Check sheet for the modelled part. Datum: model origin and axes. Units: mm. Face numbers are marked on the shaded views. A direction names the side the tool comes from. Round coordinates to 2 decimals unless told otherwise and drop trailing zeros. Order: outer loops, then holes, each group sorted by start corner. A loop starts at its lowest first (then second) coordinate and runs counter-clockwise, first axis right, second up. Notation, with made-up numbers: (-3, 63) -> (50, 63) arc R29 cw to (50, 89) -> close; hole circle Ø1 at (-22, 18). An arc over 180 degrees is marked (long way). Answer in a Markdown table with one row per item.
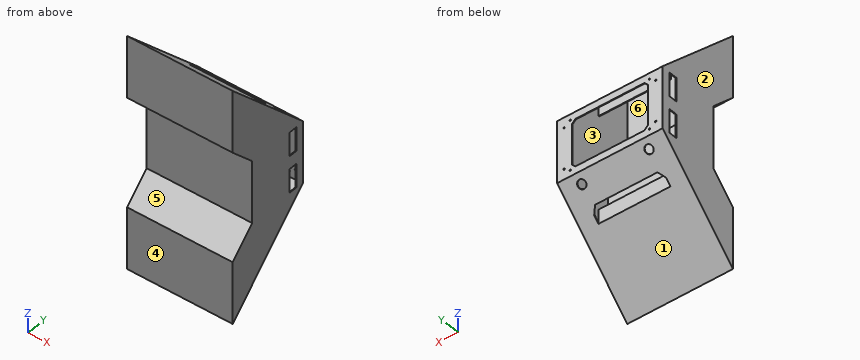
```python
from build123d import *

# Parameters (mm, degrees)
SKETCH1_W                = 220
SKETCH1_H                = 130.5
BOSS_EXTRUDE1_DEPTH      = 3
SKETCH5_W                = 220
SKETCH5_H                = 130.5
BOSS_EXTRUDE2_DEPTH      = 127
SKETCH6_W                = 220
SKETCH6_H                = 130.5
BOSS_EXTRUDE3_DEPTH      = 1
BOSS_EXTRUDE4_DEPTH      = 110
BOSS_EXTRUDE4_DEPTH_BACK = 110
SHELL2_START             = -108.5
SHELL2_DEPTH             = 217
SKETCH2_R                = 1.5
CUT_EXTRUDE1_DEPTH       = 3
CUT_EXTRUDE2_DEPTH       = 10
CUT_EXTRUDE3_DEPTH       = 322.833128344
CUT_EXTRUDE3_DEPTH_BACK  = 322.833128344
SKETCH7_W                = 50
SKETCH7_H                = 18
SKETCH9_R                = 8.5
CUT_EXTRUDE4_DEPTH       = 10
CUT_EXTRUDE5_DEPTH       = 322.833128344
CUT_EXTRUDE5_DEPTH_BACK  = 322.833128344
SKETCH11_W               = 150
SKETCH11_H               = 30
BOSS_EXTRUDE5_DEPTH      = 1.5
SKETCH12_R               = 8.5
CUT_EXTRUDE6_DEPTH       = 1.5


# Read off the part's stored shape, not the designer's step: Shell2
with BuildPart() as part:
    # Sketch1 → Boss-Extrude1 (new body)
    with BuildSketch(Plane(origin=(0, 0, 0), x_dir=(1, 0, 0), z_dir=(0, 1, 0))):
        Rectangle(SKETCH1_W, SKETCH1_H)
    extrude(amount=BOSS_EXTRUDE1_DEPTH)

    # Sketch5 → Boss-Extrude2 (add)
    with BuildSketch(Plane(origin=(0, 0, 0), x_dir=(1, 0, 0), z_dir=(0, 1, 0))):
        Rectangle(SKETCH5_W, SKETCH5_H)
    extrude(amount=-BOSS_EXTRUDE2_DEPTH)

    # Sketch6 → Boss-Extrude3 (add)
    with BuildSketch(Plane.XZ.offset(127)):
        Rectangle(SKETCH6_W, SKETCH6_H)
    extrude(amount=-BOSS_EXTRUDE3_DEPTH)

    # Sketch8 → Boss-Extrude4 (add, two sides: drawn at the far end of the back side and taken through both)
    with BuildSketch(Plane(origin=(0, 0, 0), x_dir=(0, 0, -1), z_dir=(1, 0, 0)).offset(-BOSS_EXTRUDE4_DEPTH_BACK)):
        Polygon((-65.25, 3), (-65.25, -127), (-115.25, -177), (-245.25, -177), align=None)
        Polygon((245.25, -177), (65.25, 3), (65.25, -127), (115.25, -177), align=None)
    extrude(amount=BOSS_EXTRUDE4_DEPTH + BOSS_EXTRUDE4_DEPTH_BACK)

    # Shell2 outline → Shell2 (cut)
    with BuildSketch(Plane.YZ.offset(SHELL2_START)):
        Polygon((-175.5, -241.628679656), (1.5, -64.628679656), (1.5, 64.628679656), (-175.5, 241.628679656), (-175.5, 115.871320344), (-125.5, 65.871320344), (-125.5, -65.871320344), (-175.5, -115.871320344), align=None)
    extrude(amount=SHELL2_DEPTH, mode=Mode.SUBTRACT)

    # Sketch2 → Cut-Extrude1 (cut)
    with BuildSketch(Plane(origin=(0, 0, 0), x_dir=(1, 0, 0), z_dir=(0, 1, 0))):
        with Locations(Location((-82.5, 52.5, 0), (0, 0, 270))):
            Circle(SKETCH2_R)
        with Locations(Location((-82.5, -52.5, 0), (0, 0, 90))):
            Circle(SKETCH2_R)
        with Locations(Location((82.5, -52.5, 0), (0, 0, 270))):
            Circle(SKETCH2_R)
        with Locations(Location((82.5, 52.5, 0), (0, 0, 90))):
            Circle(SKETCH2_R)
        with Locations(Location((-95.5, 43.5, 0), (0, 0, 270))):
            Circle(SKETCH2_R)
        with Locations(Location((-95.5, -43.5, 0), (0, 0, 90))):
            Circle(SKETCH2_R)
        with Locations(Location((95.5, -43.5, 0), (0, 0, 270))):
            Circle(SKETCH2_R)
        with Locations(Location((95.5, 43.5, 0), (0, 0, 90))):
            Circle(SKETCH2_R)
    extrude(amount=CUT_EXTRUDE1_DEPTH, mode=Mode.SUBTRACT)

    # Sketch4 → Cut-Extrude2 (cut)
    with BuildSketch(Plane(origin=(0, 0, 0), x_dir=(1, 0, 0), z_dir=(0, 1, 0))):
        Polygon((-79, 42.928932188), (-71.928932188, 50), (71.928932188, 50), (79, 42.928932188), (79, -42.928932188), (71.928932188, -50), (-71.928932188, -50), (-79, -42.928932188), align=None)
    extrude(amount=CUT_EXTRUDE2_DEPTH, mode=Mode.SUBTRACT)

    # Sketch7 → Cut-Extrude3 (cut, two sides: drawn at the far end of the back side and taken through both)
    with BuildSketch(Plane(origin=(0, 0, 0), x_dir=(0, 0, -1), z_dir=(1, 0, 0)).offset(-CUT_EXTRUDE3_DEPTH_BACK)):
        with Locations((-38.5, -23)):
            Rectangle(SKETCH7_W, SKETCH7_H)
        with Locations((38.5, -23)):
            Rectangle(SKETCH7_W, SKETCH7_H)
    extrude(amount=CUT_EXTRUDE3_DEPTH + CUT_EXTRUDE3_DEPTH_BACK, mode=Mode.SUBTRACT)

    # Sketch9 → Cut-Extrude4 (cut)
    with BuildSketch(Plane(origin=(0, 34.125, 34.125), x_dir=(1, 0, 0), z_dir=(0, 0.7071067811865435, 0.7071067811865517))):
        with Locations(Location((70, -64.017397129, 0), (0, 0, 270))):
            Circle(SKETCH9_R)
        with Locations(Location((-70, -64.017397129, 0), (0, 0, 270))):
            Circle(SKETCH9_R)
    extrude(amount=-CUT_EXTRUDE4_DEPTH, mode=Mode.SUBTRACT)

    # Sketch10 → Cut-Extrude5 (cut, two sides: drawn at the far end of the back side and taken through both)
    with BuildSketch(Plane.XY.offset(-CUT_EXTRUDE5_DEPTH_BACK)):
        Polygon((-75, -49), (-65, -39), (65, -39), (75, -49), (75, -60.2132), (-75, -60.2132), align=None)
    extrude(amount=CUT_EXTRUDE5_DEPTH + CUT_EXTRUDE5_DEPTH_BACK, mode=Mode.SUBTRACT)

    # Sketch11 → Boss-Extrude5 (add)
    with BuildSketch(Plane(origin=(0, -60.2132, 0), x_dir=(1, 0, 0), z_dir=(0, 1, 0))):
        with Locations((0, -113.4632)):
            Rectangle(SKETCH11_W, SKETCH11_H)
        with Locations((0, 113.4632)):
            Rectangle(SKETCH11_W, SKETCH11_H)
    extrude(amount=-BOSS_EXTRUDE5_DEPTH)

    # Sketch12 → Cut-Extrude6 (cut)
    with BuildSketch(Plane(origin=(0, 19.989962184, -48.260037816), x_dir=(1, 0, 0), z_dir=(0, -0.7071067811865438, 0.7071067811865513))):
        with Locations(Location((70, -44.027434945, 0), (0, 0, 270))):
            Circle(SKETCH12_R)
        with Locations(Location((-70, -44.027434945, 0), (0, 0, 90))):
            Circle(SKETCH12_R)
    extrude(amount=CUT_EXTRUDE6_DEPTH, mode=Mode.SUBTRACT)


solid = part.part
```
(1) Draft check along X on the marked faces 1, 2 and 3. Enter one of: pulls with the +X half, pulls with the -X half, needs draft (parallel to the pull), parting line crosses it, or undercut.
Solutions:
| item | result |
|---|---|
| face 1 | needs draft |
| face 2 | pulls with the -X half |
| face 3 | undercut |
(2) Tool access check on the marked faces 4, 5 and 6. Record the directions out of +Z, -Z, +X, -X, +Y, -Y that give a thin tool (end or side, any length) a straight path to the whole face; none if there is none.
Solutions:
| item | result |
|---|---|
| face 4 | +Z, -Z, +X, -X, -Y |
| face 5 | +X, -X, -Y |
| face 6 | none |
(3) Section check C-C on z = 215.5. Record the boundary of the cut face in (x, y), plus the area to 3 significant figures.
Solutions:
| item | result |
|---|---|
| outline | (-110, -177) -> (110, -177) -> (110, -147.25) -> (-110, -147.25) -> close; hole (-108.5, -175.5) -> (108.5, -175.5) -> (108.5, -149.37) -> (-108.5, -149.37) -> close |
| area | 875 mm^2 |
(4) Section check A-A on z = -31. Record the boundary of the cut face in (x, y).
Solutions:
| item | result |
|---|---|
| outline | (-110, -127) -> (110, -127) -> (110, -32) -> (108.5, -32) -> (108.5, -125.5) -> (-108.5, -125.5) -> (-108.5, -32) -> (-110, -32) -> close; (-110, -14) -> (-108.5, -14) -> (-108.5, 1.5) -> (-79, 1.5) -> (-79, 3) -> (-110, 3) -> close; (79, 1.5) -> (108.5, 1.5) -> (108.5, -14) -> (110, -14) -> (110, 3) -> (79, 3) -> close |
(5) Section check D-D on y = -90.5. Record the boundary of the cut face in (x, z), plus the area to 3 significant figures.
Solutions:
| item | result |
|---|---|
| outline | (-110, -158.75) -> (110, -158.75) -> (110, 158.75) -> (-110, 158.75) -> close; hole (-108.5, -156.63) -> (108.5, -156.63) -> (108.5, 156.63) -> (-108.5, 156.63) -> close |
| area | 1,870 mm^2 |
(6) Section check B-B on x = 9.5. Give the number of separate pieces and of enclosed holes in the cut face, plus the area to 3 significant figures.
Solutions:
| item | result |
|---|---|
| separate pieces | 3 |
| enclosed holes | 0 |
| area | 1,590 mm^2 |
(7) Scan lines: probe 1 along X at (y, z) = (2.05, 43.5); probe 2 along X at (y, z) = (2, -43); probe 3 along X at (y, z) = (2, -52). Record each from-to range of solid material in increasing order. Write a range as from..to.
Solutions:
| item | result |
|---|---|
| probe 1 | -110..-97, -94..-78.43, 78.43..94, 97..110 |
| probe 2 | -110..-96.91, -94.09..-78.93, 78.93..94.09, 96.91..110 |
| probe 3 | -110..-83.91, -81.09..81.09, 83.91..110 |
(8) Depth check by flat-ended pin: pin 1 Ø12 at (x, z) = (-83, 131.5) entering from +Y; pin 2 Ø1.2 at (x, y) = (-109.5, -24.5) entering from +Z; pin 3 Ø8 at (x, z) = (-43.5, -47) entering from -Y. Enter the tip coordinate at first touch or a pass-through.
Solutions:
| item | result |
|---|---|
| pin 1 | y = -57.25 |
| pin 2 | z = 93.35 |
| pin 3 | y = -127 |
